Could you check a few things on this model? Use its own coordinates, in mm. Face numbers are marked on the shaded views. A direction names the side the tool comes from. Give positions to 0.01 mm unless a question says otherwise; leave off trailing zeros. Order: outer loops, then holes, each group sorted by start corner. A loop starts at its lowest first (then second) coordinate and runs counter-clockwise, first axis right, second up. Notation, with made-up numbers: (-10.5, 50.5) -> (7.5, 50.5) arc R17 cw to (7.5, 55.5) -> close; hole circle Ø7 at (48.25, 29.5). An arc over 180 degrees is marked (long way). Answer as CSV lines item,"result". Start each with the question number.
(1) I want a section at D-D (y = -8.75). Please give me the cut outline in (x, z).
(2) Will these pins go through, and if not, where does the flat tip stop? pin 1 Ø2.5 at (x, z) = (18.5, 35) entering from -Y; pin 2 Ø0.8 at (x, y) = (19, -1.5) entering from +Z; pin 3 Ø0.8 at (x, y) = (19, -2.5) entering from -Z; pin 4 Ø4.5 at (x, z) = (19, 12) entering from -Y.
(3) We'd pull the mould along Z, two halves only. Please class the marked faces 1, 2 and 3: released by +Z, released by -Z, zero draft, split by the parting line, or undercut.
(4) I want a section at A-A (x = -16). Please give me the cut outline in (y, z), plus the area to 3 significant figures.
(5) On a 3-axis mill with a long thin cutter (end or side, diameter ignored), from which of +Z, -Z, +X, -X, +Y, -Y can I reach the whole of each face in a straight line? I mean the marked faces 4, 5 and 6. Say none if no direction works.
(6) I want a section at B-B (z = 40.5). Please give me the cut outline in (x, y), plus the area to 3 significant figures.
(7) I need wall thicknesses on L1, parallel to X at y = -1.8, z = 35; L2, parallel to X at y = -3.9, z = 12; L3, parallel to X at y = -0.75, z = 8.5. Which ranges of each line are inside material? Lowest first, please.
(8) I want a section at C-C (x = 20.5). Please give me the cut outline in (y, z).
```python
from build123d import *

# Parameters (mm, degrees)
SKETCH1_W               = 30
SKETCH1_H               = 32
SKETCH1_R               = 8.05
BOSS_EXTRUDE1_DEPTH     = 47
CUT_EXTRUDE1_DEPTH      = 52.86520992
CUT_EXTRUDE1_DEPTH_BACK = 52.86520992
SKETCH3_W               = 30
SKETCH3_H               = 16
SKETCH4_W               = 8
SKETCH4_H               = 8
SKETCH4_R               = 2.05
BOSS_EXTRUDE2_DEPTH     = 5.5
FILLET1_R               = 3.5


with BuildPart() as part:
    # Sketch1 → Boss-Extrude1 (new body)
    with BuildSketch(Plane.XY):
        Rectangle(SKETCH1_W, SKETCH1_H)
        Circle(SKETCH1_R, mode=Mode.SUBTRACT)
    extrude(amount=BOSS_EXTRUDE1_DEPTH)

    # Sketch3 → Cut-Extrude1 (cut, two sides: drawn at the far end of the back side and taken through both)
    with BuildSketch(Plane.XY.offset(-CUT_EXTRUDE1_DEPTH_BACK)):
        with Locations((0, 8)):
            Rectangle(SKETCH3_W, SKETCH3_H)
    extrude(amount=CUT_EXTRUDE1_DEPTH + CUT_EXTRUDE1_DEPTH_BACK, mode=Mode.SUBTRACT)

    # Sketch4 → Boss-Extrude2 (add)
    # profile 1 of 4: a face of its own
    with BuildSketch(Plane(origin=(0, 0, 0), x_dir=(1, 0, 0), z_dir=(0, 1, 0))):
        with Locations((19, -12)):
            Rectangle(SKETCH4_W, SKETCH4_H)
        with Locations(Location((19, -12, 0), (0, 0, 270))):
            Circle(SKETCH4_R, mode=Mode.SUBTRACT)
    # profile 2 of 4: a face of its own
    with BuildSketch(Plane(origin=(0, 0, 0), x_dir=(1, 0, 0), z_dir=(0, 1, 0))):
        with Locations((-19, -35)):
            Rectangle(SKETCH4_W, SKETCH4_H)
        with Locations(Location((-19, -35, 0), (0, 0, 270))):
            Circle(SKETCH4_R, mode=Mode.SUBTRACT)
    # profile 3 of 4: a face of its own
    with BuildSketch(Plane(origin=(0, 0, 0), x_dir=(1, 0, 0), z_dir=(0, 1, 0))):
        with Locations((19, -35)):
            Rectangle(SKETCH4_W, SKETCH4_H)
        with Locations(Location((19, -35, 0), (0, 0, 90))):
            Circle(SKETCH4_R, mode=Mode.SUBTRACT)
    # profile 4 of 4: a face of its own
    with BuildSketch(Plane(origin=(0, 0, 0), x_dir=(1, 0, 0), z_dir=(0, 1, 0))):
        with Locations((-19, -12)):
            Rectangle(SKETCH4_W, SKETCH4_H)
        with Locations(Location((-19, -12, 0), (0, 0, 90))):
            Circle(SKETCH4_R, mode=Mode.SUBTRACT)
    extrude(amount=-BOSS_EXTRUDE2_DEPTH)

    # Fillet1
    fillet1_edges = [part.edges().sort_by_distance(p)[0] for p in [
        (-23, -2.75, 8),
        (-15, -2.75, 8),
        (-15, -2.75, 16),
        (-23, -2.75, 16),
        (23, -2.75, 39),
        (15, -2.75, 39),
        (15, -2.75, 31),
        (23, -2.75, 31),
        (-15, -2.75, 31),
        (-15, -2.75, 39),
        (-23, -2.75, 39),
        (-23, -2.75, 31),
        (15, -2.75, 16),
        (15, -2.75, 8),
        (23, -2.75, 8),
        (23, -2.75, 16),
    ]]
    fillet(fillet1_edges, radius=FILLET1_R)


solid = part.part
```
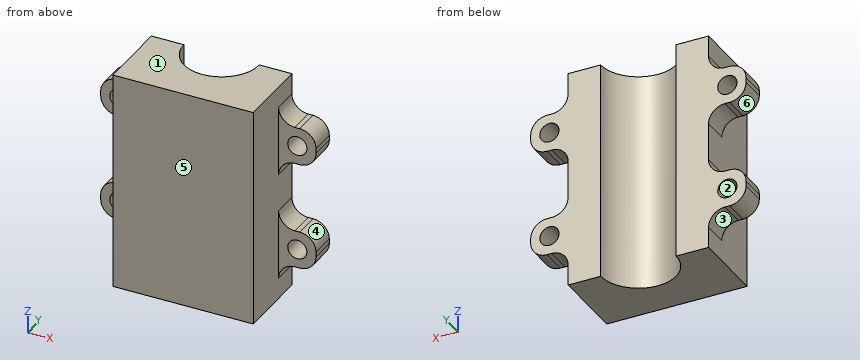
Final values:
1,outline,"(-15, 0) -> (15, 0) -> (15, 47) -> (-15, 47) -> close"
2,pin 1,"through"
2,pin 2,"z = 39"
2,pin 3,"z = 8"
2,pin 4,"y = -5.5"
3,face 1,"released by +Z"
3,face 2,"undercut"
3,face 3,"released by -Z"
4,outline,"(-5.5, 6.95) -> (0, 6.95) -> (0, 17.05) -> (-5.5, 17.05) -> close; (-5.5, 29.95) -> (0, 29.95) -> (0, 40.05) -> (-5.5, 40.05) -> close"
4,area,"111 mm²"
5,face 4,"+X, +Y, -Y"
5,face 5,"+Z, -Z, +X, -X, -Y"
5,face 6,"-X, +Y, -Y"
6,outline,"(-15.63, -5.5) -> (-15, -5.5) -> (-15, -16) -> (15, -16) -> (15, -5.5) -> (15.63, -5.5) -> (15.63, 0) -> (8.05, 0) arc R8.05 cw to (-8.05, 0) -> (-15.63, 0) -> close"
6,area,"385 mm²"
7,L1,"-23 to -21.05, -16.95 to -7.85, 7.85 to 16.95, 21.05 to 23"
7,L2,"-23 to -21.05, -16.95 to -7.04, 7.04 to 16.95, 21.05 to 23"
7,L3,"-21.3 to -8.01, 8.01 to 21.3"
8,outline,"(-5.5, 8.15) -> (0, 8.15) -> (0, 10.6) -> (-5.5, 10.6) -> close; (-5.5, 13.4) -> (0, 13.4) -> (0, 15.85) -> (-5.5, 15.85) -> close; (-5.5, 31.15) -> (0, 31.15) -> (0, 33.6) -> (-5.5, 33.6) -> close; (-5.5, 36.4) -> (0, 36.4) -> (0, 38.85) -> (-5.5, 38.85) -> close"
